Autodesk Inventor part; units mm, degrees
ref_plane "YZ Plane" through (0, 0, 0) normal (1, 0, 0) x (0, 1, 0)
ref_plane "XZ Plane" through (0, 0, 0) normal (0, 1, 0) x (-1, 0, 0)
ref_plane "XY Plane" through (0, 0, 0) normal (0, 0, 1) x (1, 0, 0)
sketch "Sketch1" plane through (0, 0, 0) normal (0, 1, 0) x (-1, 0, 0)
  line L0 (-30, -11.6205) -> (30, -11.6205)
  line L1 (30, -11.6205) -> (30, 11.6205)
  line L2 (30, 11.6205) -> (-30, 11.6205)
  line L3 (-30, 11.6205) -> (-30, -11.6205)
  line L4 (-30, -11.6205) -> (30, 11.6205) construction
  line L5 (30, -11.6205) -> (-30, 11.6205) construction
  line L6 (-9.746, 11.6205) -> (-9.746, 5.2705)
  line L7 (-9.746, 5.2705) -> (-30, 5.2705)
  line L8 (30, 5.2705) -> (9.746, 5.2705)
  line L9 (9.746, 5.2705) -> (9.746, 11.6205)
  line L10 (30, 0) -> (0, 0) construction
  line L11 (-9.746, -11.6205) -> (-9.746, -5.2705)
  line L12 (-9.746, -5.2705) -> (-30, -5.2705)
  line L13 (30, -5.2705) -> (9.746, -5.2705)
  line L14 (9.746, -5.2705) -> (9.746, -11.6205)
  line L15 (30, -11.6205) -> (30, -21.6205)
  line L16 (30, -21.6205) -> (-20, -50.488)
  line L17 (-20, -50.488) -> (-30, -50.488)
  line L18 (-30, -50.488) -> (-30, -11.6205)
  dimension "d0" = 20.254
  dimension "d1" = 20.254
  dimension "d2" = 6.35
  dimension "d3" = 60
  dimension "d4" = 23.241
  dimension "d5" = 10
  dimension "d6" = 10
  dimension "d7" = 60
extrude "Plate1" add sketch "Sketch1" along normal blind 4.7625 contours L0 L15 L16 L17 L18 | L11 L12 L3 L7 L6 L2 L9 L8 L1 L13 L14 L0
fillet "Corner Round1" radius 6 3 edges at (-30, 2.3813, -21.6205) (20, 2.3813, -50.488) (30, 2.3813, -50.488)
sketch "Sketch2" plane through (0, 4.7625, 0) normal (0, 1, 0) x (1, 0, 0)
  line L0 (-21.1962, 18.6205) -> (23, 18.6205)
  line L1 (23, 18.6205) -> (23, 44.1372)
  line L2 (23, 44.1372) -> (-21.1962, 18.6205)
  line L3 (-27, 23.3526) -> (18.6077, 49.6842)
  line L4 (-9.746, 11.6205) -> (-30, 11.6205)
  line L5 (30, 44.488) -> (30, 11.6205)
  point P0 (0, 0)
  dimension "d10" = 7
  dimension "d11" = 7
  dimension "d12" = 7
hole "Hole1" at (-21.1962, 4.7625, -18.6205) at (23, 4.7625, -18.6205) at (23, 4.7625, -44.1372) direction (0, -1, 0) diameter 5.105 end through all
equation "\"d1\" = d0"
equation "\"d6\" = d5"
equation "\"d11\" = d10"
equation "\"d12\" = d10"
equation "\"d18\" = Thickness"
equation "\"d8\" = Thickness"
equation "\"BendRadius\" = Thickness"
equation "\"BendReliefWidth\" = Thickness"
equation "\"BendReliefDepth\" = 0.5 * Thickness"
equation "\"CornerReliefSize\" = 4 * Thickness"
equation "\"MinimumRemnant\" = 2 * Thickness"
equation "\"TransitionRadius\" = BendRadius"
equation "\"JacobiRadiusSize\" = BendRadius"
equation "\"GapSize\" = Thickness"
properties part number "INTAKE_BACK_MOUNT_PLATE" material "Aluminum, 6061-T6"
Here's how the part is built. I have some questions about the finished solid (model axes, mm). A direction names the side the tool comes from. Round coordinates to 2 decimals unless told otherwise and drop trailing zeros. Loops run counter-clockwise (first coordinate to the right, second up) from the corner with the lowest first, then second, coordinate; pieces in that order, holes last.
1. If we section it at D-D on z = -20: Write out the boundary of the cut face in (x, y), plus the area to 3 significant figures.
Answer list:
outline: (-29.71, 0) - (-23.34, 0) - (-23.34, 4.76) - (-29.71, 4.76) - close; (-19.05, 0) - (20.85, 0) - (20.85, 4.76) - (-19.05, 4.76) - close; (25.15, 0) - (30, 0) - (30, 4.76) - (25.15, 4.76) - close
area: 243 mm2
2. If I drill on line 1 along Z through (x, y) = (23, 2.3); line 2 along Z through (x, y) = (-20, 2.5); line 3 along Z through (x, y) = (21.5, 1.8), over which ranges is the centre line in solid material (lowest first)?
Answer list:
line 1: z = -50.49 to -46.69, -41.58 to -21.17, -16.07 to -11.62, -5.27 to 5.27
line 2: z = -27.39 to -20.88, -16.37 to -11.62, -5.27 to 5.27
line 3: z = -50.49 to -46.2, -42.07 to -20.69, -16.56 to -11.62, -5.27 to 5.27
3. If we section it at B-B on y = 2.9: Write out the boundary of the cut face in (x, z) (1 decimal).
Answer list:
outline: (-30, -18.2) arc R6 ccw to (-27, -23.4) - (18.6, -49.7) arc R6 ccw to (21.6, -50.5) - (24, -50.5) arc R6 ccw to (30, -44.5) - (30, -11.6) - (9.7, -11.6) - (9.7, -5.3) - (30, -5.3) - (30, 5.3) - (9.7, 5.3) - (9.7, 11.6) - (-9.7, 11.6) - (-9.7, 5.3) - (-30, 5.3) - (-30, -5.3) - (-9.7, -5.3) - (-9.7, -11.6) - (-30, -11.6) - close; hole circle Ø5.1 at (-21.2, -18.6); hole circle Ø5.1 at (23, -44.1); hole circle Ø5.1 at (23, -18.6)
4. If we section it at A-A on x = 23: Write out the boundary of the cut face in (y, z).
Answer list:
outline: (0, -50.49) - (4.76, -50.49) - (4.76, -46.69) - (0, -46.69) - close; (0, -41.58) - (4.76, -41.58) - (4.76, -21.17) - (0, -21.17) - close; (0, -16.07) - (4.76, -16.07) - (4.76, -11.62) - (0, -11.62) - close; (0, -5.27) - (4.76, -5.27) - (4.76, 5.27) - (0, 5.27) - close
5. For P1, Ø2.5, axis at y = 2, z = -7, coming from the +X side; P2, Ø4, axis at x = -21.2, z = -18.62, coming from the -Y side; P3, Ø1.4, axis at x = -23, y = 2.5, coming from the +Z side, each with a flat end and sliding along its axis, tell me the tip position at first contact or that it passes through.
Answer list:
P1: stops at x = 9.75
P2: passes through
P3: stops at z = 5.27
6. If we section it at C-C on x = -20: Write out the boundary of the cut face in (y, z).
Answer list:
outline: (0, -27.39) - (4.76, -27.39) - (4.76, -20.88) - (0, -20.88) - close; (0, -16.37) - (4.76, -16.37) - (4.76, -11.62) - (0, -11.62) - close; (0, -5.27) - (4.76, -5.27) - (4.76, 5.27) - (0, 5.27) - close
7. We'd pull the mould along X, two halves only. Please class faces 1 (the face through (23.978, 2.348, -16.263)), 2 (the face through (22.888, 2.348, -46.687)), 3 (the face through (30, 2, 0)), 4 (the face through (-20, 2, -11.62)): +X half, -X half, draft (parallel to the pull), parting line (faces both ways), or undercut.
Answer list:
face 1: undercut
face 2: undercut
face 3: +X half
face 4: draft
8. Which directions (+Z, -Z, +X, -X, +Y, -Y) give clear straight access to the entire face, cutting with the end or side of a thin tool? Please do faces 5 (the face through (20, 2, -11.62)), 6 (the face through (20, 2, 5.27)), 7 (the face through (-20, 2, -5.27)), 8 (the face through (-20, 2, 5.27)).
Answer list:
face 5: +X, +Y, -Y
face 6: +Z, +X, +Y, -Y
face 7: -X, +Y, -Y
face 8: +Z, -X, +Y, -Y
